```python
from build123d import *

# Parameters (mm, degrees)
SKETCH1_R           = 11.1125
BOSS_EXTRUDE1_DEPTH = 3.175
CHAMFER1_SIZE       = 0.508


with BuildPart() as part:
    # Sketch1 → Boss-Extrude1 (new body)
    with BuildSketch(Plane(origin=(0, 0, 0), x_dir=(1, 0, 0), z_dir=(0, 1, 0))):
        with Locations(Location((0, 0, 0), (0, 0, 270))):
            Circle(SKETCH1_R)
        Polygon((7.552318871, 0), (3.776159436, 6.5405), (-3.776159436, 6.5405), (-7.552318871, 0), (-3.776159436, -6.5405), (3.776159436, -6.5405), align=None, mode=Mode.SUBTRACT)
    extrude(amount=BOSS_EXTRUDE1_DEPTH)

    # Chamfer1
    chamfer1_edges = [part.edges().sort_by_distance(p)[0] for p in [
        (0, 0, -6.5405),
        (-5.664239153, 0, -3.27025),
        (-5.664239153, 0, 3.27025),
        (0, 0, 6.5405),
        (5.664239153, 3.175, 3.27025),
        (5.664239153, 3.175, -3.27025),
        (0, 3.175, -6.5405),
        (-5.664239153, 3.175, -3.27025),
        (-5.664239153, 3.175, 3.27025),
        (0, 3.175, 6.5405),
        (0, 0, -11.1125),
        (0, 3.175, -11.1125),
        (5.664239153, 0, 3.27025),
        (5.664239153, 0, -3.27025),
    ]]
    chamfer(chamfer1_edges, length=CHAMFER1_SIZE)


solid = part.part
```
Could you check a few things on this model? Use its own coordinates, in mm. A direction names the side the tool comes from. Coordinates: 2 decimals unless noted, no trailing zeros. Loops run counter-clockwise (first coordinate to the right, second up) from the corner with the lowest first, then second, coordinate; pieces in that order, holes last. Notation, with made-up numbers: M 89,-24.5 L 113,-24.5 A38 cw 113,14.5 Z; hole C -33.75,-13.75 d3. An arc over 180 degrees is marked long. Put each result on its own line as item: value. Start each with the question number.
(1) I need wall thicknesses on line 1 (X direction, y = 2.1, z = 3.75); line 2 (X direction, y = 2.85, z = 2.25); line 3 (Z direction, x = 3.75, y = 2.9). Which ranges of each line are inside material? Lowest first, please. Write a range as from..to.
(2) Suppose I cut it at A-A on x = 0. Please give me the cut outline in (y, z) (1 decimal), then the cut area to 3 significant figures.
(3) For faces 4 (the face through (5.691, 1.572, -3.224)), 5 (the face through (-5.86, 0.25, -3.45)), 6 (the face through (-5.859, 2.925, -3.448)), 7 (the face through (-7, 3.175, -3)), which set-ups out of +Z, -Z, +X, -X, +Y, -Y let a thin tool reach every point of the face, with its end or its side?
(4) Thinking about a two-plate mould opening in Z: for faces 1 (the face through (5.638, 1.572, 3.316)), 2 (the face through (9.37, 1.572, 5.974)), 3 (the face through (-7, 0, -3)), which applies, pulls with the +Z half, pulls with the -Z half, needs draft (parallel to the pull), parting line crosses it, or undercut?
(5) Suppose I cut it at B-B on y = 1.35. Please give me the cut outline in (x, z) (1 decimal), then the cut area to 3 significant figures.
(6) Will these pins go through, and if not, where does the flat tip stop? P1, Ø1.5, axis at x = -5, y = 1.5, coming from the -Z side; P2, Ø1, axis at y = 2.5, z = -3, coming from the -X side; P3, Ø1, axis at y = 3, z = 4, coming from the -X side.
Solutions:
1. line 1: x = -10.46..-5.39, 5.39..10.46
1. line 2: x = -10.7..-6.46, 6.46..10.7
1. line 3: z = -10.21..-6.77, 6.77..10.21
2. outline: M 0,-10.6 L 0.5,-11.1 L 2.7,-11.1 L 3.2,-10.6 L 3.2,-7 L 2.7,-6.5 L 0.5,-6.5 L 0,-7 Z; M 0,7 L 0.5,6.5 L 2.7,6.5 L 3.2,7 L 3.2,10.6 L 2.7,11.1 L 0.5,11.1 L 0,10.6 Z
2. area: 28.0 mm2
3. face 4: +Y, -Y
3. face 5: -Y
3. face 6: +Y
3. face 7: +Z, -Z, +X, -X, +Y
4. face 1: undercut
4. face 2: parting line crosses it
4. face 3: needs draft
5. outline: C 0,0 d22.2; hole M -7.6,0 L -3.8,-6.5 L 3.8,-6.5 L 7.6,0 L 3.8,6.5 L -3.8,6.5 Z
5. area: 240 mm2
6. P1: stops at z = -10.27
6. P2: stops at x = -10.83
6. P3: stops at x = -10.5
